Autodesk Inventor part; units mm, degrees
ref_plane "YZ Plane" through (0, 0, 0) normal (1, 0, 0) x (0, 1, 0)
ref_plane "XZ Plane" through (0, 0, 0) normal (0, 1, 0) x (-1, 0, 0)
ref_plane "XY Plane" through (0, 0, 0) normal (0, 0, 1) x (1, 0, 0)
sketch "スケッチ1" plane through (0, 0, 0) normal (0, 0, 1) x (1, 0, 0)
  line L0 (14, 22.5) -> (-14, 22.5)
  line L1 (-16, 20.5) -> (-16, -20.5)
  line L2 (-14, -22.5) -> (14, -22.5)
  line L3 (16, -20.5) -> (16, 20.5)
  line L4 (16, 22.5) -> (-16, -22.5) construction
  line L5 (-16, 22.5) -> (16, -22.5) construction
  line L6 (-13, 19.5) -> (13, 19.5) construction
  line L7 (13, 19.5) -> (13, -19.5) construction
  line L8 (13, -19.5) -> (-13, -19.5) construction
  line L9 (-13, -19.5) -> (-13, 19.5) construction
  line L10 (-13, 19.5) -> (13, -19.5) construction
  line L11 (13, 19.5) -> (-13, -19.5) construction
  circle A0 centre (-13, -19.5) radius 1.1
  line L12 (-16, 0) -> (16, 0) construction
  line L13 (0, 22.5) -> (0, -22.5) construction
  circle A1 centre (-13, 19.5) radius 1.1
  circle A2 centre (13, -19.5) radius 1.1
  circle A3 centre (13, 19.5) radius 1.1
  circle A4 centre (-13, -19.5) radius 2 construction
  circle A5 centre (-13, 19.5) radius 2 construction
  circle A6 centre (13, -19.5) radius 2 construction
  circle A7 centre (13, 19.5) radius 2 construction
  circle A8 centre (0, 0) radius 7.25
  arc A9 (-16, -20.5) -> (-14, -22.5) centre (-14, -20.5) ccw
  arc A10 (14, -22.5) -> (16, -20.5) centre (14, -20.5) ccw
  arc A11 (16, 20.5) -> (14, 22.5) centre (14, 20.5) ccw
  arc A12 (-14, 22.5) -> (-16, 20.5) centre (-14, 20.5) ccw
  line L14 (-10.5, 11.5) -> (10.5, 11.5)
  line L15 (11.5, 10.5) -> (11.5, -10.5)
  line L16 (10.5, -11.5) -> (-10.5, -11.5)
  line L17 (-11.5, -10.5) -> (-11.5, 10.5)
  line L18 (-11.5, 11.5) -> (11.5, -11.5) construction
  line L19 (11.5, 11.5) -> (-11.5, -11.5) construction
  line L20 (3.85, -24.5) -> (-3.85, -24.5)
  line L21 (-3.85, -24.5) -> (-3.85, -15.5)
  line L22 (-3.85, -15.5) -> (3.85, -15.5)
  line L23 (3.85, -15.5) -> (3.85, -24.5)
  line L24 (3.85, -24.5) -> (-3.85, -15.5) construction
  line L25 (-3.85, -24.5) -> (3.85, -15.5) construction
  line L26 (-4.5, 21.5) -> (4.5, 21.5)
  line L27 (4.5, 21.5) -> (4.5, 15)
  line L28 (4.5, 15) -> (-4.5, 15)
  line L29 (-4.5, 15) -> (-4.5, 21.5)
  line L30 (-4.5, 21.5) -> (4.5, 15) construction
  line L31 (4.5, 21.5) -> (-4.5, 15) construction
  arc A13 (-10.5, 11.5) -> (-11.5, 10.5) centre (-10.5, 10.5) ccw
  arc A14 (-11.5, -10.5) -> (-10.5, -11.5) centre (-10.5, -10.5) ccw
  arc A15 (10.5, -11.5) -> (11.5, -10.5) centre (10.5, -10.5) ccw
  arc A16 (11.5, 10.5) -> (10.5, 11.5) centre (10.5, 10.5) ccw
  arc A17 (-12.5, 2) -> (-12.5, -2) centre (-12.5, 0) ccw
  line L32 (-12.5, 2) -> (-11.5, 2)
  line L33 (-12.5, -2) -> (-11.5, -2)
  arc A18 (12.5, -2) -> (12.5, 2) centre (12.5, 0) ccw
  line L34 (12.5, 2) -> (11.5, 2)
  line L35 (12.5, -2) -> (11.5, -2)
  point P0 (0, -20)
  point P1 (0, 18.25)
  point P2 (3.85, -22.5)
  point P3 (-3.85, -22.5)
  dimension "d0" = 32
  dimension "d1" = 45
  dimension "d5" = 2.2
  dimension "d6" = 4
  dimension "d34" = 2
  dimension "d40" = 26
  dimension "d41" = 39
  dimension "d42" = 14.5
  dimension "d43" = 23
  dimension "d44" = 23
  dimension "d45" = 7.7
  dimension "d46" = 9
  dimension "d47" = 2
  dimension "d48" = 9
  dimension "d49" = 6.5
  dimension "d50" = 1
  dimension "d57" = 1
  dimension "d58" = 2
  dimension "d59" = 1
extrude "押し出し1" add sketch "スケッチ1" along normal blind 1.6 contours A11 L3 A10 L2 L23 L22 L21 A9 L1 A12 L0 | L2 L21 L22 L23 | A8 | L14 A16 L15 A15 L16 A14 L17 A13 | L17 L33 A17 L32 | L34 A18 L35 L15 | L26 L27 L28 L29
extrude "押し出し2" add sketch "スケッチ1" along normal blind 6.1 contours L14 A16 L15 A15 L16 A14 L17 A13 | L17 L33 A17 L32 | L34 A18 L35 L15
extrude "押し出し3" add sketch "スケッチ1" along normal blind 18 contours A8
extrude "押し出し4" add sketch "スケッチ1" along normal blind 5.5 contours L23 L20 L21 L2 | L2 L21 L22 L23
extrude "押し出し5" cut sketch "スケッチ1" along normal blind 1.6 contours L23 L20 L21 L2
extrude "押し出し6" add sketch "スケッチ1" along normal blind 5.3 contours L26 L27 L28 L29
properties part number "KBCR-S02MU"
Design review of the part built by this model. Coordinates are the model's own, in mm. A direction names the side the tool comes from. Round coordinates to 2 decimals unless told otherwise and drop trailing zeros. Order: outer loops, then holes, each group sorted by start corner. A loop starts at its lowest first (then second) coordinate and runs counter-clockwise, first axis right, second up. Notation, with made-up numbers: (52, -28.75) - (76, -28.75) arc R21 ccw to (76, -13.75) - close; hole circle Ø5 at (52.25, 79.5). An arc over 180 degrees is marked (long way). One line per question, with ' | ' between items.
Item 1: Machinability: for faces 1 (the face through (-11.199, -11.215, 3.818)), 2 (the face through (11.215, -11.199, 3.818)), 3 (the face through (-11.5, 6, 4)), 4 (the face through (14.5, 0, 3.8)), which of the approach directions +Z, -Z, +X, -X, +Y, -Y give a long, thin tool a straight path to every point of the face, cutting with its end or side? Answer none if there is none.
Checks:
face 1: +Z, -X, -Y | face 2: +Z, +X, -Y | face 3: +Z, -X, +Y | face 4: +Z, +X
Item 2: Take a section at B-B, the plane y = -19.5. Write out the cut boundary in (x, z), then the cut area to 3 significant figures.
Checks:
outline: (-16, 0) - (-14.1, 0) - (-14.1, 1.6) - (-16, 1.6) - close; (-11.9, 0) - (11.9, 0) - (11.9, 1.6) - (3.85, 1.6) - (3.85, 5.5) - (-3.85, 5.5) - (-3.85, 1.6) - (-11.9, 1.6) - close; (14.1, 0) - (16, 0) - (16, 1.6) - (14.1, 1.6) - close | area: 74.2 mm²
Item 3: Wall thickness on line 1 (Y direction, x = 13, z = 0.8); line 2 (Z direction, x = 5, y = 17); line 3 (X direction, y = 0, z = 3): over which ranges is each line inside the solid? List them lowest first. Write a range as [from, to].
Checks:
line 1: [-22.5, -20.6], [-18.4, 18.4], [20.6, 22.5] | line 2: [0, 1.6] | line 3: [-14.5, 14.5]
Item 4: Take a section at A-A, the plane z = 3. Write out the cut boundary in (x, y).
Checks:
outline: (-12.5, -2) - (-11.5, -2) - (-11.5, -10.5) arc R1 ccw to (-10.5, -11.5) - (10.5, -11.5) arc R1 ccw to (11.5, -10.5) - (11.5, -2) - (12.5, -2) arc R2 ccw to (12.5, 2) - (11.5, 2) - (11.5, 10.5) arc R1 ccw to (10.5, 11.5) - (-10.5, 11.5) arc R1 ccw to (-11.5, 10.5) - (-11.5, 2) - (-12.5, 2) arc R2 ccw to start; (-4.5, 15) - (4.5, 15) - (4.5, 21.5) - (-4.5, 21.5) - close; (-3.85, -24.5) - (3.85, -24.5) - (3.85, -15.5) - (-3.85, -15.5) - close
Item 5: Draft analysis for pull direction Y (two halves, no side actions). For faces 5 (the face through (0, 11.5, 4)), 6 (the face through (0, 0, 0)), 7 (the face through (12.762, 20.574, 0.789)), 8 (the face through (11.199, 11.215, 3.818)), state which applies: +Y half, -Y half, draft (parallel to the pull), parting line (faces both ways), or undercut.
Checks:
face 5: undercut | face 6: draft | face 7: undercut | face 8: +Y half
Item 6: Take a section at D-D, the plane y = 0. Write out the cut boundary in (x, z).
Checks:
outline: (-16, 0) - (16, 0) - (16, 1.6) - (14.5, 1.6) - (14.5, 6.1) - (7.25, 6.1) - (7.25, 18) - (-7.25, 18) - (-7.25, 6.1) - (-14.5, 6.1) - (-14.5, 1.6) - (-16, 1.6) - close
Item 7: For P1, Ø1, axis at y = -17.5, z = 2.5, coming from the -X side; P2, Ø3.5, axis at x = -13, y = 19.5, coming from the +Z side; P3, Ø1.3, axis at y = 8, z = 3.5, coming from the +X side, all flat-tipped, find the tip position at first contact; note any pin that passes through.
Checks:
P1: x = -3.85 | P2: z = 1.6 | P3: x = 11.5
Item 8: Take a section at C-C, the plane x = 0. Write out the cut boundary in (y, z), then the cut area to 3 significant figures.
Checks:
outline: (-24.5, 1.6) - (-22.5, 1.6) - (-22.5, 0) - (22.5, 0) - (22.5, 1.6) - (21.5, 1.6) - (21.5, 5.3) - (15, 5.3) - (15, 1.6) - (11.5, 1.6) - (11.5, 6.1) - (7.25, 6.1) - (7.25, 18) - (-7.25, 18) - (-7.25, 6.1) - (-11.5, 6.1) - (-11.5, 1.6) - (-15.5, 1.6) - (-15.5, 5.5) - (-24.5, 5.5) - close | area: 407 mm²
